Input: part model. Units: mm. Frame: model coordinates. Coordinates: 2 decimals unless noted, no trailing zeros. Write each loop counter-clockwise with the first axis right and the second up, starting at its lowest first coordinate (ties: lowest second). Pieces come first, ordered by that corner, then holes.
Autodesk Inventor part; units mm, degrees
ref_plane "YZ Plane" through (0, 0, 0) normal (1, 0, 0) x (0, 1, 0)
ref_plane "XZ Plane" through (0, 0, 0) normal (0, 1, 0) x (-1, 0, 0)
ref_plane "XY Plane" through (0, 0, 0) normal (0, 0, 1) x (1, 0, 0)
sketch "Sketch1" plane through (0, 0, 0) normal (0, 0, 1) x (1, 0, 0)
  point P0 (0, 0)
sketch "Sketch2" plane through (0, 0, 0) normal (0, 0, 1) x (1, 0, 0)
  line L0 (0, 0) -> (99.06, 0)
  line L1 (99.06, 0) -> (99.06, 15.24)
  line L2 (99.06, 15.24) -> (0, 15.24)
  line L3 (0, 15.24) -> (0, 0)
  dimension "d0" = 15.24
  dimension "d1" = 99.06
extrude "Extrusion1" add sketch "Sketch2" along normal blind 2.032
sketch "Sketch3" plane through (0, 0, 2.032) normal (0, 0, 1) x (1, 0, 0)
  line L0 (0, 15.24) -> (0, 0)
  line L1 (0, 7.62) -> (99.06, 7.62)
  line L2 (99.06, 0) -> (99.06, 15.24)
  point P0 (12.7, 7.62)
  dimension "d14" = 12.7
hole "Hole1" at (12.7, 7.62, 2.032) direction (0, 0, -1) diameter 7.62 end through all
pattern_linear "Rectangular Pattern1" count 5 spacing 15.24 along (1, 0, 0) of "Hole1"
sketch "Sketch4" plane through (0, 0, 2.032) normal (0, 0, 1) x (1, 0, 0)
  line L0 (99.06, 0) -> (99.06, 15.24)
  line L1 (99.06, 7.62) -> (91.44, 7.62)
  point P0 (0, 0)
  dimension "d15" = 7.62
hole "Hole2" at (91.44, 7.62, 2.032) direction (0, 0, -1) diameter 2.54 end through all
sketch "Sketch5" plane through (0, 0, 2.032) normal (0, 0, 1) x (1, 0, 0)
  line L0 (0, 0) -> (83.82, 0)
  line L1 (83.82, 0) -> (83.82, 2.54)
  line L2 (83.82, 2.54) -> (0, 2.54)
  line L3 (0, 2.54) -> (0, 0)
  dimension "d23" = 83.82
  dimension "d24" = 2.54
extrude "Extrusion2" add sketch "Sketch5" along normal blind 2.032
fillet "Fillet1" radius 5.08 2 edges at (99.06, 15.24, 1.016) (99.06, 0, 1.016)
fillet "Fillet2" radius 2.54 2 edges at (0, 15.24, 1.016) (0, 0, 2.032)
equation "\"d15\" = 0.5 * d0"
properties part number "Lopez_LeftLeg" material "Polypropylene"
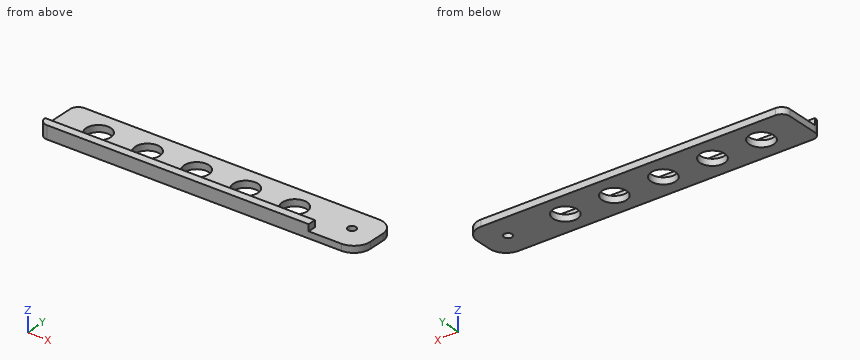
Item 1: Section query D-D, the plane x = 79.5. Return loops of the section in (y, z).
Item 2: Material intervals for line 1 (Y direction, x = 43.18, z = 0.7); line 2 (X direction, y = 10.75, z = 1); line 3 (Z direction, x = 69, y = 7.25), sorted ascending.
Item 3: Pin query (flat end, axial travel): pin 1 Ø1 at (x, z) = (44, 3.5) entering from +Y; pin 2 Ø2 at (y, z) = (1, 3.5) entering from +X; pin 3 Ø4.5 at (x, y) = (33, 7) entering from +Z. Return the tip coordinate at first contact, or that it passes through.
Item 4: Section query C-C, the plane z = 1.2. Return loops of the section in (x, y), then the cut area to 3 significant figures.
Item 5: Section query A-A, the plane x = 27.94. Return loops of the section in (y, z), then the cut area to 3 significant figures.
Item 6: Section query B-B, the plane y = 7.62. Return loops of the section in (x, z), then the cut area to 3 significant figures.
The answers:
1. outline: (0, 0) - (15.24, 0) - (15.24, 2.03) - (2.54, 2.03) - (2.54, 4.06) - (0, 4.06) - close
2. line 1: y = 0 to 3.81, 11.43 to 15.24
2. line 2: x = 0 to 10.53, 14.87 to 25.77, 30.11 to 41.01, 45.35 to 56.25, 60.59 to 71.49, 75.83 to 99.03
2. line 3: z = 0 to 2.03
3. pin 1: stops at y = 2.54
3. pin 2: stops at x = 83.82
3. pin 3: stops at z = 2.03
4. outline: (0, 2.54) arc R2.54 ccw to (2.54, 0) - (93.98, 0) arc R5.08 ccw to (99.06, 5.08) - (99.06, 10.16) arc R5.08 ccw to (93.98, 15.24) - (2.54, 15.24) arc R2.54 ccw to (0, 12.7) - close; hole circle Ø7.62 at (12.7, 7.62); hole circle Ø7.62 at (27.94, 7.62); hole circle Ø7.62 at (43.18, 7.62); hole circle Ø7.62 at (58.42, 7.62); hole circle Ø7.62 at (73.66, 7.62); hole circle Ø2.54 at (91.44, 7.62)
4. area: 1,260 mm2
5. outline: (0, 0) - (3.81, 0) - (3.81, 2.03) - (2.54, 2.03) - (2.54, 4.06) - (0, 4.06) - close; (11.43, 0) - (15.24, 0) - (15.24, 2.03) - (11.43, 2.03) - close
5. area: 20.6 mm2
6. outline: (0, 0) - (8.89, 0) - (8.89, 2.03) - (0, 2.03) - close; (16.51, 0) - (24.13, 0) - (24.13, 2.03) - (16.51, 2.03) - close; (31.75, 0) - (39.37, 0) - (39.37, 2.03) - (31.75, 2.03) - close; (46.99, 0) - (54.61, 0) - (54.61, 2.03) - (46.99, 2.03) - close; (62.23, 0) - (69.85, 0) - (69.85, 2.03) - (62.23, 2.03) - close; (77.47, 0) - (90.17, 0) - (90.17, 2.03) - (77.47, 2.03) - close; (92.71, 0) - (99.06, 0) - (99.06, 2.03) - (92.71, 2.03) - close
6. area: 119 mm2
